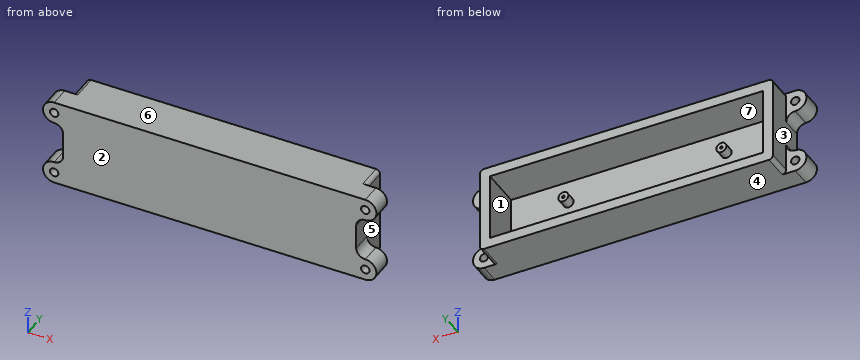
```python
from build123d import *

# Parameters (mm, degrees)
SKETCH1_W                 = 172.7
SKETCH1_H                 = 42.7
SKETCH1_R                 = 3.175
BOSS_EXTRUDE1_DEPTH       = 3.175
BOSS_EXTRUDE2_START       = 3.175
SKETCH1_3_R               = 3.175
BOSS_EXTRUDE2_DEPTH       = 6.35
SKETCH1_4_W               = 185.4
SKETCH1_4_H               = 55.4
SKETCH1_4_W_2             = 172.7
SKETCH1_4_H_2             = 42.7
BOSS_EXTRUDE3_DEPTH       = 28.575
SKETCH1_5_R               = 2.667
BOSS_EXTRUDE4_DEPTH       = 12.7
M2X0_4_TAPPED_HOLE1_D     = 1.6
M2X0_4_TAPPED_HOLE1_DEPTH = 5.19938
M2X0_4_TAPPED_HOLE1_TIP   = 0.480688495
FILLET1_R                 = 2.54


with BuildPart() as part:
    # Sketch1 → Boss-Extrude1 (new body)
    with BuildSketch(Plane(origin=(0, 0, 0), x_dir=(1, 0, 0), z_dir=(0, 1, 0))):
        with Locations((92.7, 27.7)):
            Rectangle(SKETCH1_W, SKETCH1_H)
        with Locations((142.7, 20.7)):
            Circle(SKETCH1_R, mode=Mode.SUBTRACT)
        with Locations((42.7, 20.7)):
            Circle(SKETCH1_R, mode=Mode.SUBTRACT)
        with Locations((42.7, 20.7)):
            Circle(SKETCH1_R)
        with Locations((142.7, 20.7)):
            Circle(SKETCH1_R)
    extrude(amount=BOSS_EXTRUDE1_DEPTH)

    # Sketch1<3> → Boss-Extrude2 (add)
    with BuildSketch(Plane(origin=(0, 0, 0), x_dir=(1, 0, 0), z_dir=(0, 1, 0)).offset(BOSS_EXTRUDE2_START)):
        with Locations((42.7, 20.7)):
            Circle(SKETCH1_3_R)
        with Locations((142.7, 20.7)):
            Circle(SKETCH1_3_R)
    extrude(amount=BOSS_EXTRUDE2_DEPTH)

    # Sketch1<4> → Boss-Extrude3 (add)
    with BuildSketch(Plane(origin=(0, 0, 0), x_dir=(1, 0, 0), z_dir=(0, 1, 0))):
        with Locations((92.7, 27.7)):
            Rectangle(SKETCH1_4_W, SKETCH1_4_H)
        with Locations((92.7, 27.7)):
            Rectangle(SKETCH1_4_W_2, SKETCH1_4_H_2, mode=Mode.SUBTRACT)
    extrude(amount=BOSS_EXTRUDE3_DEPTH)

    # Sketch1<5> → Boss-Extrude4 (add)
    with BuildSketch(Plane(origin=(0, 0, 0), x_dir=(1, 0, 0), z_dir=(0, 1, 0))):
        with BuildLine():
            Line((-5.725, 0), (0, 0))
            Line((0, 0), (0, 19.85))
            ThreePointArc((0, 19.85), (-1.676813678, 15.801813678), (-5.725, 14.125))
            ThreePointArc((-5.725, 14.125), (-12.7875, 7.0625), (-5.725, 0))
        make_face()
        with Locations((-5.725, 7.0625)):
            Circle(SKETCH1_5_R, mode=Mode.SUBTRACT)
        with BuildLine():
            ThreePointArc((-5.725, 41.275), (-1.676813678, 39.598186322), (0, 35.55))
            Line((0, 35.55), (0, 55.4))
            Line((0, 55.4), (-5.725, 55.4))
            ThreePointArc((-5.725, 55.4), (-12.7875, 48.3375), (-5.725, 41.275))
        make_face()
        with Locations((-5.725, 48.3375)):
            Circle(SKETCH1_5_R, mode=Mode.SUBTRACT)
        with BuildLine():
            Line((185.4, 19.85), (185.4, 0))
            Line((185.4, 0), (191.125, 0))
            ThreePointArc((191.125, 0), (198.1875, 7.0625), (191.125, 14.125))
            ThreePointArc((191.125, 14.125), (187.076813678, 15.801813678), (185.4, 19.85))
        make_face()
        with Locations((191.125, 7.0625)):
            Circle(SKETCH1_5_R, mode=Mode.SUBTRACT)
        with BuildLine():
            Line((185.4, 55.4), (185.4, 35.55))
            ThreePointArc((185.4, 35.55), (187.076813678, 39.598186322), (191.125, 41.275))
            ThreePointArc((191.125, 41.275), (198.1875, 48.3375), (191.125, 55.4))
            Line((191.125, 55.4), (185.4, 55.4))
        make_face()
        with Locations((191.125, 48.3375)):
            Circle(SKETCH1_5_R, mode=Mode.SUBTRACT)
    extrude(amount=BOSS_EXTRUDE4_DEPTH)

    # M2x0.4 Tapped Hole1
    with Locations(Plane(origin=(0, 9.525, 0), x_dir=(1, 0, 0), z_dir=(0, 1, 0))):
        with Locations((42.7, 20.7), (142.7, 20.7)):
            Hole(M2X0_4_TAPPED_HOLE1_D / 2, depth=M2X0_4_TAPPED_HOLE1_DEPTH)
            with Locations((0, 0, -(M2X0_4_TAPPED_HOLE1_DEPTH + M2X0_4_TAPPED_HOLE1_TIP / 2))):  # 118° drill point
                Cone(0, M2X0_4_TAPPED_HOLE1_D / 2, M2X0_4_TAPPED_HOLE1_TIP, mode=Mode.SUBTRACT)

    # Fillet1
    fillet1_edges = [part.edges().sort_by_distance(p)[0] for p in [
        (0, 20.6375, -55.4),
        (185.4, 20.6375, -55.4),
        (185.4, 20.6375, 0),
        (0, 20.6375, 0),
    ]]
    fillet(fillet1_edges, radius=FILLET1_R)


solid = part.part
```
Model file for the job. Use its own axes, mm. Face numbers are marked on the shaded views. A direction names the side the tool comes from. Give positions to 0.01 mm unless a question says otherwise; leave off trailing zeros. Order: outer loops, then holes, each group sorted by start corner. A loop starts at its lowest first (then second) coordinate and runs counter-clockwise, first axis right, second up.
1) Mould opens along Z. For the marked faces 4, 5, 6 and 7 say: +Z half, -Z half, draft (parallel to the pull), parting line (faces both ways), or undercut.
2) Saw through at A-A, the plane y = 24. Write the cut outline in (x, z).
3) Saw through at C-C, the plane z = -38.5. Write the cut outline in (x, y) (3 decimals), then the cut area to 3 significant figures.
4) Pin check, flat tips, straight feed: pin 1 (4.5 mm diameter, centred on x = -5.72, z = -7.06, fed in from -Y); pin 2 (8.5 mm diameter, centred on x = 191.12, z = -7.06, fed in from +Y); pin 3 (8.5 mm diameter, centred on y = 13.5, z = -25.5, fed in from +X); pin 4 (4 mm diameter, centred on x = 104, z = -10.5, fed in from +Y) (3 decimals). Stop position of each tip, or through.
5) Wall check: probe 1 along Z at (x, y) = (42.7, 7.55) (3 decimals); probe 2 along Z at (x, y) = (33.5, 23.75); probe 3 along X at (y, z) = (15, -30). Give the ranges that are in metal, low to high.
6) 3-axis set-ups, long thin cutter, end or side, ignore diameter. For the marked faces 1, 2 and 3: which of +Z, -Z, +X, -X, +Y, -Y reach the whole face in a straight line?
7) Saw through at B-B, the plane x = 131. Write the cut outline in (y, z) (3 decimals).
Computed:
1. face 4: -Z half
1. face 5: undercut
1. face 6: +Z half
1. face 7: undercut
2. outline: (0, -52.86) arc R2.54 ccw to (2.54, -55.4) - (182.86, -55.4) arc R2.54 ccw to (185.4, -52.86) - (185.4, -2.54) arc R2.54 ccw to (182.86, 0) - (2.54, 0) arc R2.54 ccw to (0, -2.54) - close; hole (6.35, -49.05) - (179.05, -49.05) - (179.05, -6.35) - (6.35, -6.35) - close
3. outline: (-0.819, 0) - (186.219, 0) - (186.219, 12.7) - (185.4, 12.7) - (185.4, 28.575) - (179.05, 28.575) - (179.05, 3.175) - (6.35, 3.175) - (6.35, 28.575) - (0, 28.575) - (0, 12.7) - (-0.819, 12.7) - close
3. area: 932 mm2
4. pin 1: passes through
4. pin 2: stops at y = 12.7
4. pin 3: stops at x = 185.4
4. pin 4: stops at y = 3.175
5. probe 1: z = -55.4 to -49.05, -23.875 to -21.5, -19.9 to -17.525, -6.35 to 0
5. probe 2: z = -55.4 to -49.05, -6.35 to 0
5. probe 3: x = 0 to 6.35, 179.05 to 185.4
6. face 1: +Y
6. face 2: +Z, -Z, +X, -X, -Y
6. face 3: -X, +Y
7. outline: (0, -55.4) - (28.575, -55.4) - (28.575, -49.05) - (3.175, -49.05) - (3.175, -6.35) - (28.575, -6.35) - (28.575, 0) - (0, 0) - close
